```python
from build123d import *

# Parameters (mm, degrees)
BOSS_EXTRUDE1_DEPTH      = 13.97
SKETCH3_W                = 1.016
SKETCH3_H                = 3.81
CUT_EXTRUDE1_DEPTH       = 14.97
CUT_EXTRUDE2_DEPTH       = 2.27
BOSS_EXTRUDE3_DEPTH      = 8.89
BOSS_EXTRUDE3_DEPTH_BACK = 25.4
SKETCH12_W               = 18.294327288
SKETCH12_H               = 7.62
BOSS_EXTRUDE4_DEPTH      = 1.27


with BuildPart() as part:
    # Sketch1 → Boss-Extrude1 (new body)
    with BuildSketch(Plane.XY):
        Polygon((0, 0), (0, 20.32), (-12.7, 20.32), (-12.7, 0), (-14.605, 0), (-14.605, 25.4), (1.905, 25.4), (1.905, 0), align=None)
    extrude(amount=-BOSS_EXTRUDE1_DEPTH)

    # Sketch3 → Cut-Extrude1 (cut, through all)
    with BuildSketch(Plane.XY):
        with Locations((-0.508, 22.225)):
            Rectangle(SKETCH3_W, SKETCH3_H)
    extrude(amount=-CUT_EXTRUDE1_DEPTH, mode=Mode.SUBTRACT)

    # Sketch4 → Cut-Extrude2 (cut, through all)
    with BuildSketch(Plane.XZ.offset(-24.13)):
        Polygon((-1.016, -6.985), (-1.016, -3.175), (0, -3.175), (0, -13.97), (-1.016, -13.97), align=None)
    extrude(amount=-CUT_EXTRUDE2_DEPTH, mode=Mode.SUBTRACT)

    # Sketch11 → Boss-Extrude3 (add, two sides)
    with BuildSketch(Plane(origin=(0, 25.4, 0), x_dir=(1, 0, 0), z_dir=(0, 1, 0))) as boss_extrude3_sk:
        Polygon((-15.497163644, 13.97), (-14.605, 13.97), (-14.605, 11.43), (-16.51, 11.43), (-16.51, 22.86), (3.81, 22.86), (3.81, 11.43), (1.905, 11.43), (1.905, 13.97), (2.797163644, 13.97), (2.797163644, 21.59), (-15.497163644, 21.59), align=None)
    extrude(amount=BOSS_EXTRUDE3_DEPTH)
    extrude(boss_extrude3_sk.sketch, amount=-BOSS_EXTRUDE3_DEPTH_BACK)

    # Sketch12 → Boss-Extrude4 (add)
    with BuildSketch(Plane.XZ):
        with Locations((-6.35, -17.78)):
            Rectangle(SKETCH12_W, SKETCH12_H)
    extrude(amount=-BOSS_EXTRUDE4_DEPTH)


solid = part.part
```
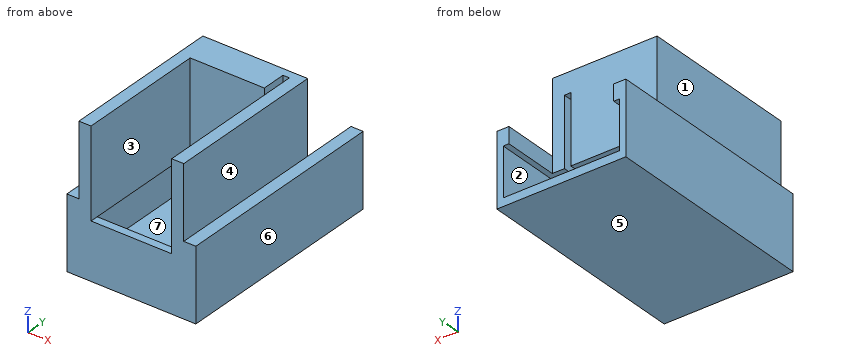
Here's how the part is built. I have some questions about the finished solid (model axes, mm). Face numbers are marked on the shaded views. A direction names the side the tool comes from. Round coordinates to 2 decimals unless told otherwise and drop trailing zeros. Order: outer loops, then holes, each group sorted by start corner. A loop starts at its lowest first (then second) coordinate and runs counter-clockwise, first axis right, second up. Notation, with made-up numbers: M -21.75,9 L -14.75,9 A31 ccw -14.75,46 Z; hole C 70,56.25 d7. An arc over 180 degrees is marked long. Use CSV: the item, a comma, the result in double quotes.
1) I want a section at D-D (z = -18.75). List the corners of the cut face in (x, y) for me.
Taken from the geometry:
outline,"M -16.51,0 L 3.81,0 L 3.81,34.29 L 2.8,34.29 L 2.8,1.27 L -15.5,1.27 L -15.5,34.29 L -16.51,34.29 Z"
2) I'm going to push flat-ended pins straight in: P1, Ø2, axis at x = 3, y = 20, coming from the +Z side; P2, Ø1.5, axis at y = 24, z = -9, coming from the +X side (3 decimals); P3, Ø3.5, axis at y = 14.5, z = -4, coming from the -X side (3 decimals); P4, Ø5, axis at y = 28.5, z = -5, coming from the -X side. Where does each tip first touch, or does it pass through?
Taken from the geometry:
P1,"z = -11.43"
P2,"x = 1.905"
P3,"x = -14.605"
P4,"through"
3) If we mould it in two halves opening along Z, with no side actions, what happens to the marked faces 5, 6 and 7? For each: pulls with the +Z half, pulls with the -Z half, needs draft (parallel to the pull), parting line crosses it, or undercut.
Taken from the geometry:
face 5,"pulls with the -Z half"
face 6,"needs draft"
face 7,"undercut"
4) I want a section at B-B (z = -13.5). List the corners of the cut face in (x, y) for me (3 decimals), then the cut area to 3 significant figures.
Taken from the geometry:
outline,"M -16.51,0 L -12.7,0 L -12.7,20.32 L -1.016,20.32 L -1.016,25.4 L -14.605,25.4 L -14.605,34.29 L -16.51,34.29 Z; M 0,0 L 3.81,0 L 3.81,34.29 L 1.905,34.29 L 1.905,25.4 L 0,25.4 Z"
area,"287 mm^2"
5) I want a section at A-A (x = -0.5). List the corners of the cut face in (y, z) for me (3 decimals), then the cut area to 3 significant figures.
Taken from the geometry:
outline,"M 0,-22.86 L 34.29,-22.86 L 34.29,-21.59 L 1.27,-21.59 L 1.27,-13.97 L 0,-13.97 Z; M 24.13,-3.175 L 25.4,-3.175 L 25.4,0 L 24.13,0 Z"
area,"57.3 mm^2"
6) On a 3-axis mill with a long thin cutter (end or side, diameter ignored), from which of +Z, -Z, +X, -X, +Y, -Y can I reach the whole of each face in a straight line? I mean the marked faces 1, 2, 3 and 4. Say none if no direction works.
Taken from the geometry:
face 1,"+Z, -X, +Y, -Y"
face 2,"+Y"
face 3,"+Z, -Y"
face 4,"+Z, +X, +Y, -Y"
7) I want a section at C-C (x = -4.25). List the corners of the cut face in (y, z) for me, then the cut area to 3 significant figures.
Taken from the geometry:
outline,"M 0,-22.86 L 34.29,-22.86 L 34.29,-21.59 L 1.27,-21.59 L 1.27,-13.97 L 0,-13.97 Z; M 20.32,-13.97 L 25.4,-13.97 L 25.4,0 L 20.32,0 Z"
area,"124 mm^2"
8) I need wall thicknesses on line 1 along Z through (x, y) = (-14.25, 5); line 2 along X through (y, z) = (2, -16); line 3 along X through (y, z) = (12, -12). Which ranges of each line are inside material? Lowest first, please. Write a range as [from, to].
Taken from the geometry:
line 1,"[-22.86, -21.59], [-13.97, 0]"
line 2,"[-16.51, -15.5], [2.8, 3.81]"
line 3,"[-16.51, -12.7], [0, 3.81]"
